Answer from the drawing. Dimensions are ordinates in mm from the lowest x, y and z of the part. A direction names the side the tool comes from. Give positions to 0.01 mm unless a question says otherwise; leave off trailing zeros. Loops run counter-clockwise (first coordinate to the right, second up) from the corner with the lowest first, then second, coordinate; pieces in that order, holes last. Notation, with made-up numbers: M -10,15.25 L 10,15.25 A28 cw 10,46.25 Z; hole C -36,13.5 d2. An arc over 180 degrees is marked long. Return JSON: item names as keys, results as strings. Group by question number.
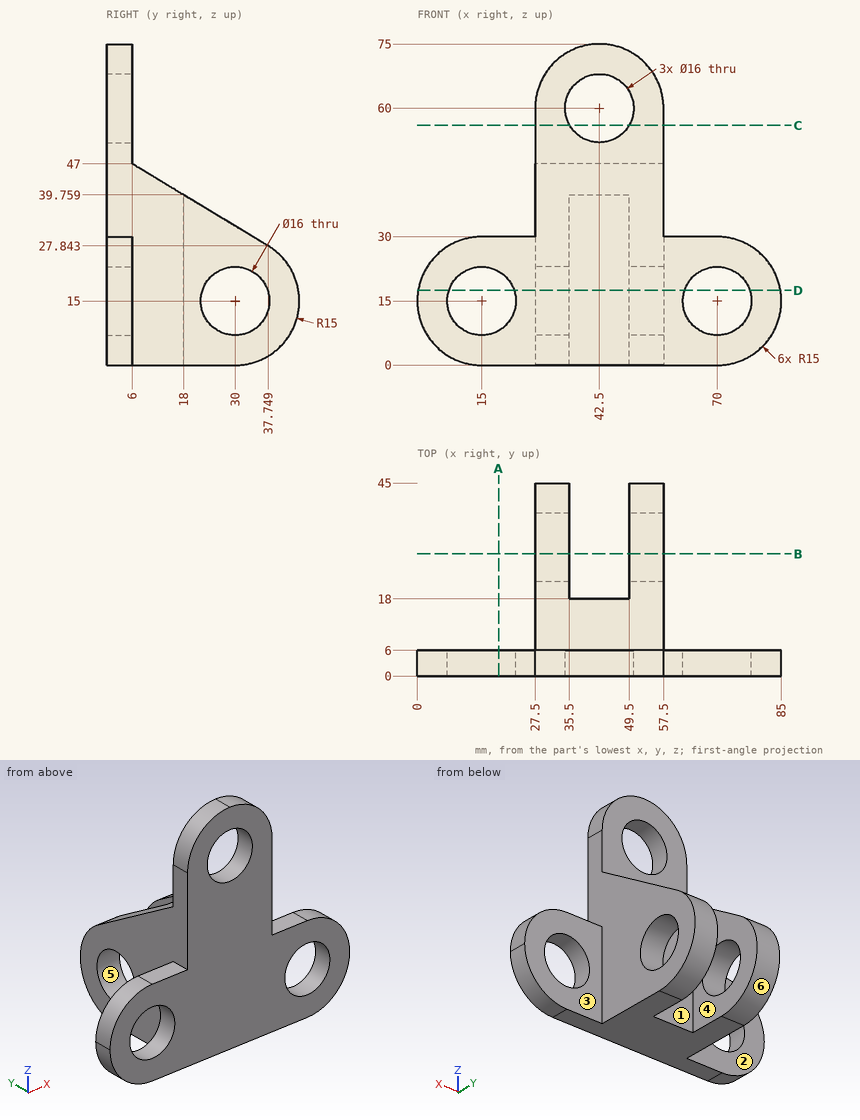
1. Straight lines are drawn through the part: line 1 along Z through (x, y) = (70, 4); line 2 along Y through (x, z) = (30, 15); line 3 along X through (y, z) = (2, 8.5) (1 decimal). For each, find the intervals that lie inside material, in ascending order.
2. Find section B-B (y = 28.5). Write down the section's boundary in (x, z) (1 decimal).
3. Find section C-C (z = 56). Write down the section's boundary in (x, y).
4. Flat-ended cylindrical pins translate along their axes: P1, Ø14, axis at x = 65.5, z = 17.5, coming from the +Y side; P2, Ø1.8, axis at x = 65, y = 2.5, coming from the +Z side; P3, Ø2, axis at y = 16.5, z = 31.5, coming from the -X side; P4, Ø9.5, axis at x = 70, z = 15, coming from the +Y side. Find the tip coordinate at first contact, or state that the pin passes through.
5. The mould has two halves that part along Z. Classify the marked faces 4, 5 and 6: +Z half, -Z half, draft (parallel to the pull), parting line (faces both ways), or undercut.
6. Find section A-A (x = 19). Write down the section's boundary in (y, z).
7. For the marked faces 1, 2 and 3, determine the directions among +Z, -Z, +X, -X, +Y, -Y from which every point of the face is accessible in a straight line to the end or side of a thin tool.
8. Find section D-D (z = 17.5). Write down the section's boundary in (x, y).
Result:
{
 "1": {"line 1": "z = 0 to 7, 23 to 30", "line 2": "y = 0 to 22, 38 to 45", "line 3": "x = 1.5 to 10.3, 19.7 to 65.3, 74.7 to 83.5"},
 "2": {"outline": "M 27.5,0 L 35.5,0 L 35.5,7.1 L 27.5,7.1 Z; M 27.5,22.9 L 35.5,22.9 L 35.5,33.4 L 27.5,33.4 Z; M 49.5,0 L 57.5,0 L 57.5,7.1 L 49.5,7.1 Z; M 49.5,22.9 L 57.5,22.9 L 57.5,33.4 L 49.5,33.4 Z"},
 "3": {"outline": "M 27.5,0 L 35.57,0 L 35.57,6 L 27.5,6 Z; M 49.43,0 L 57.5,0 L 57.5,6 L 49.43,6 Z"},
 "4": {"P1": "stops at y = 6", "P2": "stops at z = 30", "P3": "stops at x = 27.5", "P4": "passes through"},
 "5": {"face 4": "draft", "face 5": "undercut", "face 6": "parting line"},
 "6": {"outline": "M 0,0 L 6,0 L 6,8.07 L 0,8.07 Z; M 0,21.93 L 6,21.93 L 6,30 L 0,30 Z"},
 "7": {"face 1": "+Z, -Z, +Y", "face 2": "+Z, -Z, -X, +Y", "face 3": "+Z, -Z, +X, +Y"},
 "8": {"outline": "M 0.21,0 L 7.4,0 L 7.4,6 L 0.21,6 Z; M 22.6,0 L 62.4,0 L 62.4,6 L 57.5,6 L 57.5,22.4 L 49.5,22.4 L 49.5,18 L 35.5,18 L 35.5,22.4 L 27.5,22.4 L 27.5,6 L 22.6,6 Z; M 27.5,37.6 L 35.5,37.6 L 35.5,44.79 L 27.5,44.79 Z; M 49.5,37.6 L 57.5,37.6 L 57.5,44.79 L 49.5,44.79 Z; M 77.6,0 L 84.79,0 L 84.79,6 L 77.6,6 Z"}
}
